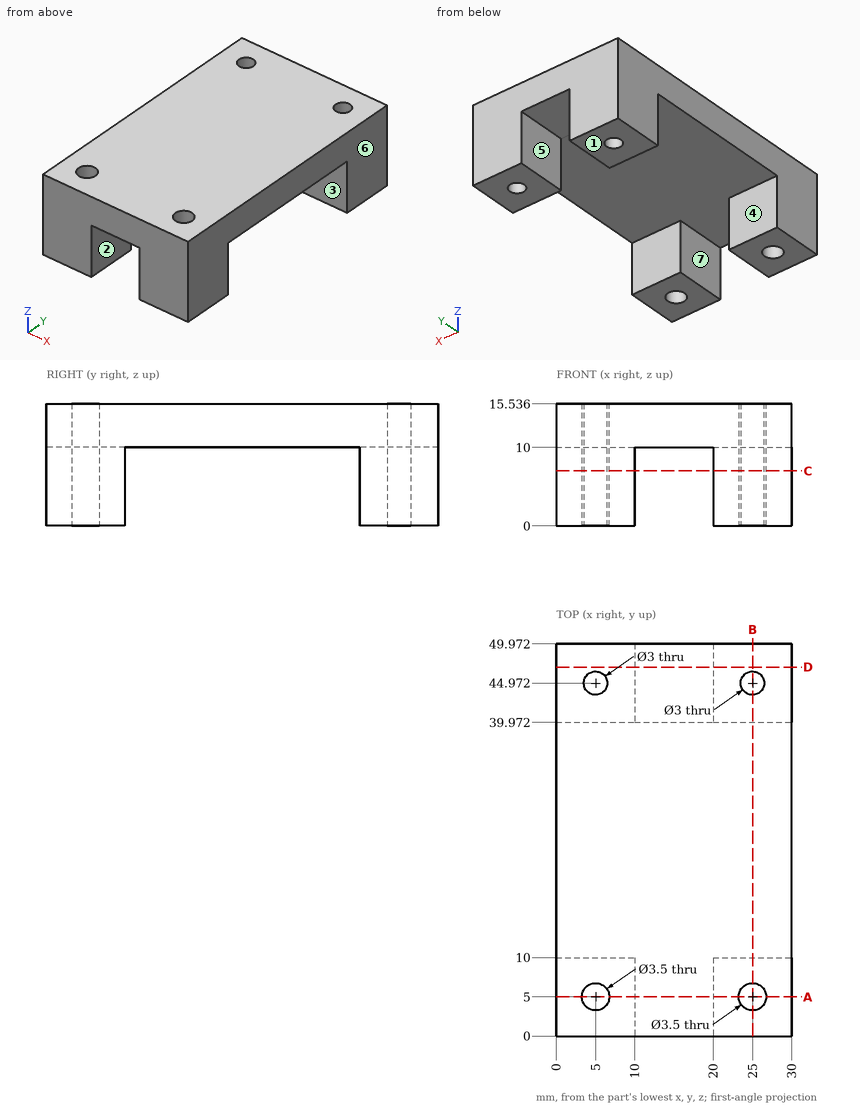
Answer from the drawing. Dimensions are ordinates in mm from the lowest x, y and z of the part. A direction names the side the tool comes from. Coordinates: 2 decimals unless noted, no trailing zeros. Write each loop counter-clockwise with the first axis right and the second up, starting at its lowest first coordinate (ties: lowest second). Pieces come first, ordered by that corner, then holes. Notation, with made-up numbers: (-13, 32.25) - (3, 32.25) arc R12 ccw to (3, 36.25) - close; hole circle Ø8 at (2.25, 51). An arc over 180 degrees is marked (long way). Return JSON: item names as keys, results as strings. Group by question number.
Q1. The part is cut by section C-C on z = 7. Write down the section's boundary in (x, y).
Q2. Find the intervals of material crossed by line 1 along Y through (x, z) = (5, 7); line 2 along X through (y, z) = (5, 12.25); line 3 along X through (y, z) = (5, 5.5), in increasing order. Write a range as [from, to].
Q3. For a pull along X with two mould halves and no side action, classify the marked faces 4, 5, 6 and 7 as +X half, -X half, draft (parallel to the pull), parting line (faces both ways), or undercut.
Q4. The part is cut by section D-D on y = 47. Write down the section's boundary in (x, z), and give its area (3 significant figures).
Q5. The part is cut by section B-B on x = 25. Write down the section's boundary in (y, z), and give its area (3 significant figures).
Q6. Which of the six approach directions +Z, -Z, +X, -X, +Y, -Y give full straight-line access (tool end or side, diameter ignored) to the marked faces 1, 2 and 3?
Q7. The part is cut by section A-A on y = 5. Write down the section's boundary in (x, z), and give its area (3 significant figures).
Q8. Flat-ended cylindrical pins translate along their axes: pin 1 Ø4 at (y, z) = (42, 11.5) entering from -X; pin 2 Ø3 at (x, y) = (5, 5) entering from +Z; pin 3 Ø9 at (x, y) = (17, 24.5) entering from -Z. Find the tip coordinate at first contact, or state that the pin passes through.
Evaluation:
{
 "1": {"outline": "(0, 0) - (10, 0) - (10, 10) - (0, 10) - close; (0, 39.97) - (10, 39.97) - (10, 49.97) - (0, 49.97) - close; (20, 0) - (30, 0) - (30, 10) - (20, 10) - close; (20, 39.97) - (30, 39.97) - (30, 49.97) - (20, 49.97) - close; hole circle Ø3.5 at (5, 5); hole circle Ø3 at (5, 44.97); hole circle Ø3.5 at (25, 5); hole circle Ø3 at (25, 44.97)"},
 "2": {"line 1": "y = [0, 3.25], [6.75, 10], [39.97, 43.47], [46.47, 49.97]", "line 2": "x = [0, 3.25], [6.75, 23.25], [26.75, 30]", "line 3": "x = [0, 3.25], [6.75, 10], [20, 23.25], [26.75, 30]"},
 "3": {"face 4": "draft", "face 5": "undercut", "face 6": "+X half", "face 7": "undercut"},
 "4": {"outline": "(0, 0) - (10, 0) - (10, 10) - (20, 10) - (20, 0) - (30, 0) - (30, 15.54) - (0, 15.54) - close", "area": "366 mm2"},
 "5": {"outline": "(0, 0) - (3.25, 0) - (3.25, 15.54) - (0, 15.54) - close; (6.75, 0) - (10, 0) - (10, 10) - (39.97, 10) - (39.97, 0) - (43.47, 0) - (43.47, 15.54) - (6.75, 15.54) - close; (46.47, 0) - (49.97, 0) - (49.97, 15.54) - (46.47, 15.54) - close", "area": "376 mm2"},
 "6": {"face 1": "-Z, +X, -X, +Y, -Y", "face 2": "-Z, +Y, -Y", "face 3": "-Z, +X, -X"},
 "7": {"outline": "(0, 0) - (3.25, 0) - (3.25, 15.54) - (0, 15.54) - close; (6.75, 0) - (10, 0) - (10, 10) - (20, 10) - (20, 0) - (23.25, 0) - (23.25, 15.54) - (6.75, 15.54) - close; (26.75, 0) - (30, 0) - (30, 15.54) - (26.75, 15.54) - close", "area": "257 mm2"},
 "8": {"pin 1": "stops at x = 0", "pin 2": "passes through", "pin 3": "stops at z = 10"}
}
